Here's how the part is built. I have some questions about the finished solid (model axes, mm). A direction names the side the tool comes from. Coordinates: 2 decimals unless noted, no trailing zeros. Write each loop counter-clockwise with the first axis right and the second up, starting at its lowest first coordinate (ties: lowest second). Pieces come first, ordered by that corner, then holes. Notation, with made-up numbers: (-21, -29.5) -> (-6, -29.5) arc R26 cw to (-6, -14.5) -> close; hole circle Ø11 at (-1.75, 15). An arc over 180 degrees is marked (long way). Answer in a Markdown table with one row per item. Add a question column.
from build123d import *

# Parameters (mm, degrees)
SKETCH_1_R          = 50
EXTRUDE_1_DEPTH     = 20
SKETCH_2_R          = 45
SKETCH_2_R_2        = 35
CUT_EXTRUDE_1_DEPTH = 10
SKETCH_3_R          = 12.5
CUT_EXTRUDE_2_DEPTH = 74.484692283
CHAMFER_1_SIZE      = 1


with BuildPart() as part:
    # 草图1 → 凸台-拉伸1 (new body)
    with BuildSketch(Plane(origin=(0, 0, 0), x_dir=(1, 0, 0), z_dir=(0, 1, 0))):
        with Locations(Location((0, 0, 0), (0, 0, 270))):
            Circle(SKETCH_1_R)
    extrude(amount=EXTRUDE_1_DEPTH)

    # 草图2 → 切除-拉伸1 (cut)
    with BuildSketch(Plane(origin=(0, 20, 0), x_dir=(1, 0, 0), z_dir=(0, 1, 0))):
        with Locations(Location((0, 0, 0), (0, 0, 270))):
            Circle(SKETCH_2_R)
        with Locations(Location((0, 0, 0), (0, 0, 270))):
            Circle(SKETCH_2_R_2, mode=Mode.SUBTRACT)
    extrude(amount=-CUT_EXTRUDE_1_DEPTH, mode=Mode.SUBTRACT)

    # 草图3 → 切除-拉伸2 (cut, through all)
    with BuildSketch(Plane(origin=(0, 0, 0), x_dir=(1, 0, 0), z_dir=(0, 1, 0))):
        with Locations(Location((0, 0, 0), (0, 0, 270))):
            Circle(SKETCH_3_R)
    extrude(amount=CUT_EXTRUDE_2_DEPTH, mode=Mode.SUBTRACT)

    # 倒角1
    chamfer_1_edges = [part.edges().sort_by_distance(p)[0] for p in [
        (0, 0, -50),
        (0, 20, -50),
    ]]
    chamfer(chamfer_1_edges, length=CHAMFER_1_SIZE)


solid = part.part
Q1. Imagine slicing it at A-A on z = 0. Please give me the cut outline in (x, y), plus the area to 3 significant figures.
Q2. Imagine slicing it at D-D on y = 4. Please give me the cut outline in (x, z), plus the area to 3 significant figures.
Q3. If we mould it in two halves opening along X, with no side actions, what happens to faces 1 (the cylindrical face through (-17.235, 15.07, 41.569)), 2 (the cylindrical face through (-21, 15, -28)), 3 (the flat face through (-10, 0, 10)), 4 (the cylindrical face through (15.02, 9.87, 47.69))? For each: pulls with the +X half, pulls with the -X half, needs draft (parallel to the pull), parting line crosses it, or undercut.
Q4. Imagine slicing it at C-C on y = 12.5. Please give me the cut outline in (x, z), plus the area to 3 significant figures.
Q5. Imagine slicing it at B-B on x = 0. Please give me the cut outline in (y, z).
Q6. I'm going to push flat-ended pins straight in: P1, Ø8, axis at x = 9.5, y = 5.5, coming from the +Z side; P2, Ø8, axis at y = 11.5, z = -33, coming from the +X side; P3, Ø5, axis at x = 12.5, y = 7.5, coming from the +Z side; P4, Ø1, axis at x = 7, z = -13.5, coming from the -Y side. Where does each tip first touch, or does it pass through?
Q7. I need wall thicknesses on line 1 (X direction, y = 5.25, z = 0); line 2 (X direction, y = 12.5, z = 0); line 3 (Z direction, x = 17.5, y = 14.5). Which ranges of each line are inside material? Lowest first, please. Write a range as [from, to].
Q8. For faces 5 (the flat face through (-26.5, 10, 23.1)), 6 (the cylindrical face through (3.755, 9.86, 11.923)), which set-ups out of +Z, -Z, +X, -X, +Y, -Y let a thin tool reach every point of the face, with its end or its side?
Result sheet:
| question | item | result |
|---|---|---|
| 1 | outline | (-50, 1) -> (-49, 0) -> (-12.5, 0) -> (-12.5, 20) -> (-35, 20) -> (-35, 10) -> (-45, 10) -> (-45, 20) -> (-49, 20) -> (-50, 19) -> close; (12.5, 0) -> (49, 0) -> (50, 1) -> (50, 19) -> (49, 20) -> (45, 20) -> (45, 10) -> (35, 10) -> (35, 20) -> (12.5, 20) -> close |
| 1 | area | 1,300 mm^2 |
| 2 | outline | circle Ø100 at (0, 0); hole circle Ø25 at (0, 0) |
| 2 | area | 7,360 mm^2 |
| 3 | face 1 | undercut |
| 3 | face 2 | undercut |
| 3 | face 3 | needs draft |
| 3 | face 4 | parting line crosses it |
| 4 | outline | circle Ø100 at (0, 0); circle Ø70 at (0, 0); hole circle Ø90 at (0, 0); hole circle Ø25 at (0, 0) |
| 4 | area | 4,850 mm^2 |
| 5 | outline | (0, -49) -> (1, -50) -> (19, -50) -> (20, -49) -> (20, -45) -> (10, -45) -> (10, -35) -> (20, -35) -> (20, -12.5) -> (0, -12.5) -> close; (0, 12.5) -> (20, 12.5) -> (20, 35) -> (10, 35) -> (10, 45) -> (20, 45) -> (20, 49) -> (19, 50) -> (1, 50) -> (0, 49) -> close |
| 6 | P1 | stops at z = 49.7 |
| 6 | P2 | stops at x = 40.73 |
| 6 | P3 | stops at z = 48.99 |
| 6 | P4 | stops at y = 0 |
| 7 | line 1 | x = [-50, -12.5], [12.5, 50] |
| 7 | line 2 | x = [-50, -45], [-35, -12.5], [12.5, 35], [45, 50] |
| 7 | line 3 | z = [-46.84, -41.46], [-30.31, 30.31], [41.46, 46.84] |
| 8 | face 5 | +Y |
| 8 | face 6 | +Y, -Y |
